```python
from build123d import *

# Parameters (mm, degrees)
SKETCH1_R           = 19.05
SKETCH1_W           = 3.175
SKETCH1_H           = 6.35
BOSS_EXTRUDE1_DEPTH = 3.175
SKETCH2_R           = 1.27
CUT_EXTRUDE1_DEPTH  = 4.175


with BuildPart() as part:
    # Sketch1 → Boss-Extrude1 (new body)
    with BuildSketch(Plane(origin=(0, 0, 0), x_dir=(1, 0, 0), z_dir=(0, 1, 0))):
        Circle(SKETCH1_R)
        Rectangle(SKETCH1_W, SKETCH1_H, mode=Mode.SUBTRACT)
    extrude(amount=BOSS_EXTRUDE1_DEPTH)

    # Sketch2 → Cut-Extrude1 (cut, through all)
    with BuildSketch(Plane(origin=(0, 3.175, 0), x_dir=(1, 0, 0), z_dir=(0, 1, 0))):
        with Locations((10.416417342, -0.454529354)):
            Circle(SKETCH2_R)
        with Locations((-10.583582658, -0.454529354)):
            Circle(SKETCH2_R)
        with Locations((-10.583582658, 11.845470646)):
            Circle(SKETCH2_R)
        with Locations((10.416417342, 11.845470646)):
            Circle(SKETCH2_R)
    extrude(amount=-CUT_EXTRUDE1_DEPTH, mode=Mode.SUBTRACT)


solid = part.part
```
Work out the finished part from the listing and answer in its coordinate system (mm). A direction names the side the tool comes from. Give positions to 0.01 mm unless a question says otherwise; leave off trailing zeros. Loops run counter-clockwise (first coordinate to the right, second up) from the corner with the lowest first, then second, coordinate; pieces in that order, holes last. Notation, with made-up numbers: (45.5, 39.25) -> (68.5, 39.25) arc R28 cw to (68.5, 59.25) -> close; hole circle Ø9 at (70.25, 76.5). An arc over 180 degrees is marked (long way). Put each result on its own line as item: value. Start each with the question number.
Item 1: The part is cut by section A-A (x = 0). Give the vertices of the cut face in (y, z) (3 decimals).
Item 2: The part is cut by section B-B (z = 0). State how many separate pieces and enclosed holes the cut face has, then the cut area to 3 significant figures.
Item 3: The part is cut by section D-D (z = 10.5). Give the vertices of the cut face in (x, y) (3 decimals).
Item 4: Each of these flat-tipped pins is pushed along its axis until it touches: P1, Ø1, axis at x = -9.5, y = 2, coming from the +Z side; P2, Ø1.6, axis at x = 0, y = 1.5, coming from the -Z side; P3, Ø1.5, axis at x = -10, y = 3, coming from the +Z side; P4, Ø10, axis at x = 5, z = 14, coming from the -Y side. Where does it stop, or does it pass through?
Item 5: Which of the six approach directions +Z, -Z, +X, -X, +Y, -Y give full straight-line access (tool end or side, diameter ignored) to faces 4 (the face through (4, 0, 0)), 5 (the face through (1.588, 2, 0))?
Item 6: The mould has two halves that part along X. Classify faces 1 (the face through (-9.41, 1.61, 0.94)), 2 (the face through (4, 3.175, 0)), 3 (the face through (-15.12, 1.57, 11.59)): released by +X, released by -X, zero draft, split by the parting line, or undercut.
Item 7: Find the intervals of material crossed by L1, parallel to X at y = 2.9, z = 0.5; L2, parallel to Z at x = 10.5, y = 0.55; L3, parallel to Z at x = 11, y = 1.35, in increasing order. Write a range as [from, to].
Answers below:
1. outline: (0, -19.05) -> (3.175, -19.05) -> (3.175, -3.175) -> (0, -3.175) -> close; (0, 3.175) -> (3.175, 3.175) -> (3.175, 19.05) -> (0, 19.05) -> close
2. separate pieces: 4
2. enclosed holes: 0
2. area: 95.8 mm2
3. outline: (-15.895, 0) -> (15.895, 0) -> (15.895, 3.175) -> (-15.895, 3.175) -> close
4. P1: z = 16.79
4. P2: z = -19.05
4. P3: z = 16.65
4. P4: y = 0
5. face 4: +Z, -Z, +X, -X, -Y
5. face 5: +Y, -Y
6. face 1: undercut
6. face 2: zero draft
6. face 3: split by the parting line
7. L1: [-19.04, -11.85], [-9.31, -1.59], [1.59, 9.15], [11.69, 19.04]
7. L2: [-15.9, -13.11], [-10.58, -0.81], [1.72, 15.9]
7. L3: [-15.55, -12.97], [-10.72, -0.67], [1.58, 15.55]
